Can you work these out from the drawing? Everything is in mm from the part's minimum corner. A direction names the side the tool comes from. Give positions to 0.01 mm unless a question says otherwise; leave off trailing zeros. Order: outer loops, then holes, each group sorted by start corner. A loop starts at its lowest first (then second) coordinate and runs counter-clockwise, first axis right, second up. Notation, with made-up numbers: M 30.5,66 L 64.5,66 A20 cw 64.5,81 Z; hole C 51.25,38 d7. An arc over 180 degrees is marked long. Use a Markdown table: item, result. Add a question column.
Item 1: Suppose I cut it at B-B on y = 12. Write out the boundary of the cut face in (x, z).
Item 2: Suppose I cut it at D-D on x = 20.75. Write out the boundary of the cut face in (y, z).
Item 3: Suppose I cut it at C-C on z = 2.25. Write out the boundary of the cut face in (x, y), plus the area to 3 significant figures.
Item 4: Suppose I cut it at A-A on x = 3. Write out the boundary of the cut face in (y, z), plus the area to 3 significant figures.
Item 5: For the marked faces 1, 2 and 3, which set-ups out of +Z, -Z, +X, -X, +Y, -Y let a thin tool reach every point of the face, with its end or its side?
Item 6: If I drill on L1, parallel to Y at x = 25.2, z = 2.15; L2, parallel to X at y = 19.5, z = 4 (1 decimal); L3, parallel to X at y = 17, z = 11.75 (1 decimal), over which ranges is the centre line in solid material (lowest first)? Write a range as from..to.
Item 7: If we mould it in two halves opening along X, with no side actions, what happens to the marked faces 4, 5 and 6? For each: released by +X, released by -X, zero draft, split by the parting line, or undercut.
Item 8: I'm going to push flat-ended pins straight in: pin 1 Ø5.5 at (x, y) = (25.2, 12) entering from -Z; pin 2 Ø4 at (x, y) = (25.2, 3) entering from +Z; pin 3 Ø1.5 at (x, z) = (5.5, 4.5) entering from +Y. Where does each tip first touch, or does it pass through?
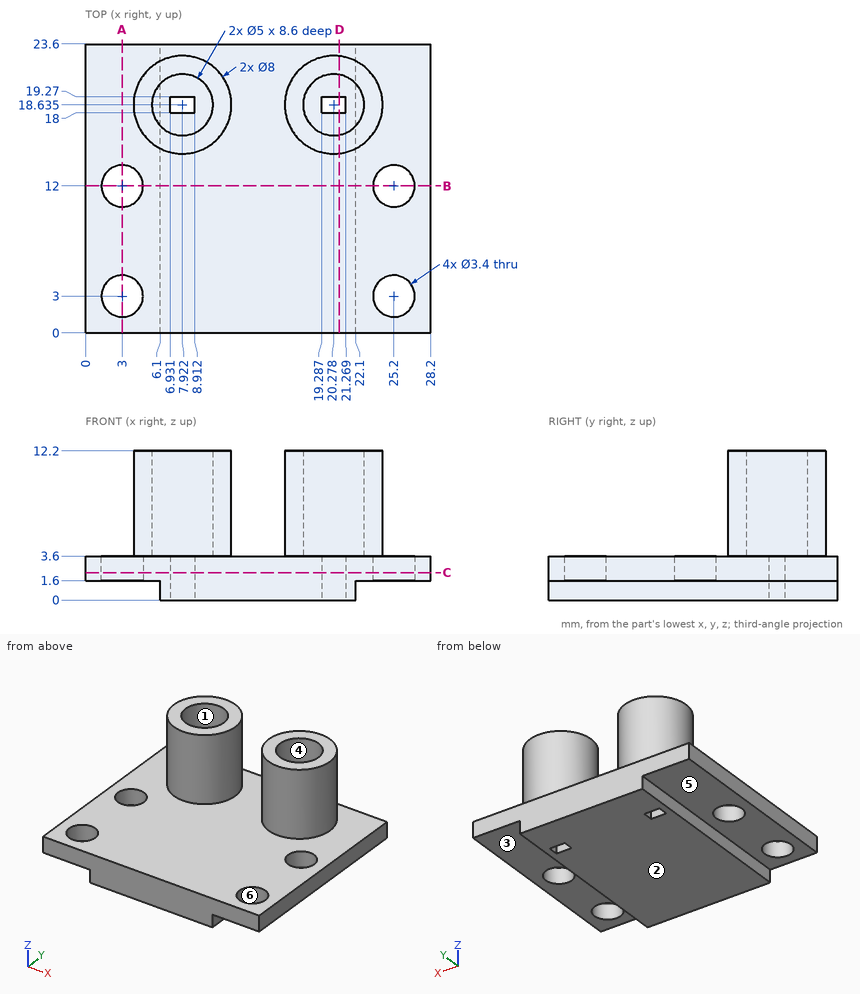
Findings below:
| question | item | result |
|---|---|---|
| 1 | outline | M 0,1.6 L 1.3,1.6 L 1.3,3.6 L 0,3.6 Z; M 4.7,1.6 L 6.1,1.6 L 6.1,0 L 22.1,0 L 22.1,1.6 L 23.5,1.6 L 23.5,3.6 L 4.7,3.6 Z; M 26.9,1.6 L 28.2,1.6 L 28.2,3.6 L 26.9,3.6 Z |
| 2 | outline | M 0,0 L 18,0 L 18,3.6 L 16.18,3.6 L 16.18,12.2 L 14.66,12.2 L 14.66,3.6 L 0,3.6 Z; M 19.27,0 L 23.6,0 L 23.6,3.6 L 22.61,3.6 L 22.61,12.2 L 21.09,12.2 L 21.09,3.6 L 19.27,3.6 Z |
| 3 | outline | M 0,0 L 28.2,0 L 28.2,23.6 L 0,23.6 Z; hole C 3,3 d3.4; hole C 3,12 d3.4; hole M 6.93,18 L 8.91,18 L 8.91,19.27 L 6.93,19.27 Z; hole M 19.29,18 L 21.27,18 L 21.27,19.27 L 19.29,19.27 Z; hole C 25.2,3 d3.4; hole C 25.2,12 d3.4 |
| 3 | area | 624 mm^2 |
| 4 | outline | M 0,1.6 L 1.3,1.6 L 1.3,3.6 L 0,3.6 Z; M 4.7,1.6 L 10.3,1.6 L 10.3,3.6 L 4.7,3.6 Z; M 13.7,1.6 L 23.6,1.6 L 23.6,3.6 L 13.7,3.6 Z |
| 4 | area | 33.6 mm^2 |
| 5 | face 1 | +Z |
| 5 | face 2 | -Z, +X, -X, +Y, -Y |
| 5 | face 3 | -Z, +X, +Y, -Y |
| 6 | L1 | y = 0..1.3, 4.7..10.3, 13.7..23.6 |
| 6 | L2 | x = 4..5.6, 10.3..11.8, 16.4..17.9, 22.6..24.2 |
| 6 | L3 | x = 4.3..6, 9.8..11.6, 16.6..18.4, 22.2..23.9 |
| 7 | face 4 | undercut |
| 7 | face 5 | zero draft |
| 7 | face 6 | undercut |
| 8 | pin 1 | stops at z = 1.6 |
| 8 | pin 2 | stops at z = 3.6 |
| 8 | pin 3 | stops at y = 22.27 |
